```python
from build123d import *

# Parameters (mm, degrees)
SKETCH2_W          = 2.5
SKETCH2_H          = 8.660254038
CUT_EXTRUDE1_DEPTH = 5


with BuildPart() as part:
    # Sketch1 → Revolve1 (revolve)
    with BuildSketch(Plane.XY):
        Polygon((-5, 5), (-5, 0), (0, 0), (0, 5), (0, 7.5), (-10, 7.5), (-10, 5), align=None)
        Polygon((50, 5), (0, 5), (0, 0), (55, 0), (55, 4.5), align=None)
    revolve(axis=Axis((0, 0, 0), (1, 0, 0)))

    # Sketch2 → Cut-Extrude1 (cut)
    with BuildSketch(Plane(origin=(55, 0, 0), x_dir=(0, 0, -1), z_dir=(1, 0, 0))):
        with Locations((-3.75, 0)):
            Rectangle(SKETCH2_W, SKETCH2_H)
        with Locations((3.75, 0)):
            Rectangle(SKETCH2_W, SKETCH2_H)
    extrude(amount=-CUT_EXTRUDE1_DEPTH, mode=Mode.SUBTRACT)


solid = part.part
```
For this review, take the finished solid that the model builds, in its own axes (mm). A direction names the side the tool comes from. Coordinates: 2 decimals unless noted, no trailing zeros. Write each loop counter-clockwise with the first axis right and the second up, starting at its lowest first coordinate (ties: lowest second). Pieces come first, ordered by that corner, then holes.
(1) Add section C-C on x = 19. Give the boundary of the cut face in (y, z).
(2) The part is to be moulded in two halves that separate along Y. For faces 6 (the face through (-5, 0, 0)), 7 (the face through (50, 0, -3)), 8 (the face through (-5.07, -7.493, 0.33)), say which applies: +Y half, -Y half, draft (parallel to the pull), parting line (faces both ways), or undercut.
(3) For pin 1 Ø1 at (x, z) = (32, 5) entering from +Y; pin 2 Ø5 at (y, z) = (-0.5, 1) entering from -X; pin 3 Ø1.3 at (y, z) = (0, 3.5) entering from +X, all flat-tipped, find the tip position at first contact; note any pin that passes through.
(4) Tool access review of faces 1 (the face through (-7.46, -1.08, -4.88)), 2 (the face through (24.65, -1.08, -4.88)), 3 (the face through (52.465, -4.753, 0.039)), 4 (the face through (53, 0, -2.5)), 5 (the face through (50, 0, 3)): name each direction out of +Z, -Z, +X, -X, +Y, -Y from which nothing blocks a thin tool from reaching the whole face with its end or side.
(5) Add section A-A on z = 0. Give the boundary of the cut face in (x, y).
(6) Add section D-D on z = 3.5. Give the boundary of the cut face in (x, y).
(7) Add section B-B on y = 0. Give the boundary of the cut face in (x, z).
(8) Wall thickness on probe 1 along Z at (x, y) = (-8.1, 0); probe 2 along X at (y, z) = (6.75, 1.25); probe 3 along X at (y, z) = (2.25, 0.5): over which ranges is each line inside the solid? List them lowest first.
Answer sheet:
1. outline: circle Ø10 at (0, 0)
2. face 6: undercut
2. face 7: draft
2. face 8: parting line
3. pin 1: stops at y = 2.18
3. pin 2: stops at x = -5
3. pin 3: stops at x = 50
4. face 1: -X
4. face 2: +X
4. face 3: +X, -Y
4. face 4: -Z, +X, +Y, -Y
4. face 5: +Z, +X, +Y, -Y
5. outline: (-10, -7.5) - (0, -7.5) - (0, -5) - (50, -5) - (55, -4.5) - (55, 4.5) - (50, 5) - (0, 5) - (0, 7.5) - (-10, 7.5) - (-10, 5) - (-5, 5) - (-5, -5) - (-10, -5) - close
6. outline: (-10, -6.63) - (0, -6.63) - (0, -3.57) - (50, -3.57) - (50, 3.57) - (0, 3.57) - (0, 6.63) - (-10, 6.63) - (-10, 3.57) - (-5, 3.57) - (-5, -3.57) - (-10, -3.57) - close
7. outline: (-10, -7.5) - (0, -7.5) - (0, -5) - (50, -5) - (50, -2.5) - (55, -2.5) - (55, 2.5) - (50, 2.5) - (50, 5) - (0, 5) - (0, 7.5) - (-10, 7.5) - (-10, 5) - (-5, 5) - (-5, -5) - (-10, -5) - close
8. probe 1: z = -7.5 to -5, 5 to 7.5
8. probe 2: x = -10 to 0
8. probe 3: x = -5 to 55
